The figure shows three views and two pictorial views of one solid part (mm, origin at its lowest corner). Answer the questions. Coordinates: 2 decimals unless noted, no trailing zeros. Order: outer loops, then holes, each group sorted by start corner. A loop starts at its lowest first (then second) coordinate and runs counter-clockwise, first axis right, second up. Notation, with made-up numbers: (-11, 63) -> (34, 63) arc R17 ccw to (34, 73) -> close; hole circle Ø7 at (-28.75, 55.25). An arc over 180 degrees is marked (long way). Write item = value, one per line. Start each with the question number.
Q1. The part is cut by section B-B, the plane x = 25. Determine the outline of the cut face in (y, z), plus the area to 3 significant figures.
Q2. For a pull along Z with two mould halves and no side action, classify the marked faces 1, 2, 3 and 4 as +Z half, -Z half, draft (parallel to the pull), parting line (faces both ways), or undercut.
Q3. The part is cut by section D-D, the plane x = 5. Determine the outline of the cut face in (y, z), plus the area to 3 significant figures.
Q4. The part is cut by section C-C, the plane y = 0.3. Determine the outline of the cut face in (x, z), plus the area to 3 significant figures.
Q5. The part is cut by section A-A, the plane z = 5. Determine the outline of the cut face in (x, y).
Q6. Straight lines are drawn through the part: L1, parallel to X at y = 0.5, z = 5; L2, parallel to X at y = 1.7, z = 5.5 (1 decimal); L3, parallel to Z at x = 23, y = 0.7. For each, find the intervals that lie inside material, in ascending order. Write a range as from..to.
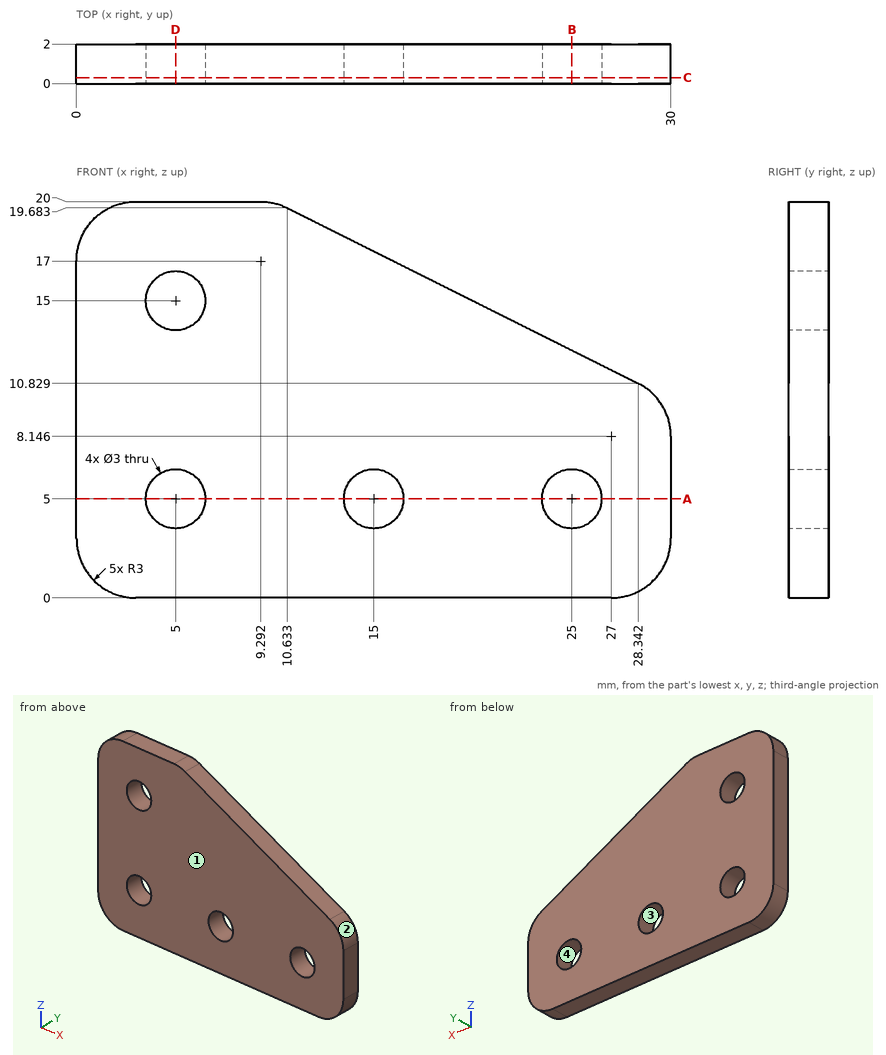
Model answer:
q1.outline = (0, 0) -> (2, 0) -> (2, 3.5) -> (0, 3.5) -> close; (0, 6.5) -> (2, 6.5) -> (2, 12.5) -> (0, 12.5) -> close
q1.area = 19.0 mm2
q2.face_1 = draft
q2.face_2 = +Z half
q2.face_3 = undercut
q2.face_4 = undercut
q3.outline = (0, 0) -> (2, 0) -> (2, 3.5) -> (0, 3.5) -> close; (0, 6.5) -> (2, 6.5) -> (2, 13.5) -> (0, 13.5) -> close; (0, 16.5) -> (2, 16.5) -> (2, 20) -> (0, 20) -> close
q3.area = 28.0 mm2
q4.outline = (0, 3) arc R3 ccw to (3, 0) -> (27, 0) arc R3 ccw to (30, 3) -> (30, 8.15) arc R3 ccw to (28.34, 10.83) -> (10.63, 19.68) arc R3 ccw to (9.29, 20) -> (3, 20) arc R3 ccw to (0, 17) -> close; hole circle Ø3 at (5, 5); hole circle Ø3 at (5, 15); hole circle Ø3 at (15, 5); hole circle Ø3 at (25, 5)
q4.area = 465 mm2
q5.outline = (0, 0) -> (3.5, 0) -> (3.5, 2) -> (0, 2) -> close; (6.5, 0) -> (13.5, 0) -> (13.5, 2) -> (6.5, 2) -> close; (16.5, 0) -> (23.5, 0) -> (23.5, 2) -> (16.5, 2) -> close; (26.5, 0) -> (30, 0) -> (30, 2) -> (26.5, 2) -> close
q6.L1 = 0..3.5, 6.5..13.5, 16.5..23.5, 26.5..30
q6.L2 = 0..3.6, 6.4..13.6, 16.4..23.6, 26.4..30
q6.L3 = 0..13.5
